```python
from build123d import *

# Parameters (mm, degrees)
F1_DEPTH = 8
F2_SIZE  = 30
F4_D     = 6.5
F6_D     = 10.5
F7_R     = 8
F8_R     = 3


with BuildPart() as f1:
    # F0 (on Front) → F1 (new body)
    with BuildSketch(Plane.XZ):
        Polygon((-41, 0), (0, 0), (0, 260), (-50, 260), (-50, 257), (-80, 257), (-80, 27), (-41, 27), align=None)
    extrude(amount=F1_DEPTH)

    # F2
    f2_edges = [f1.edges().sort_by_distance(p)[0] for p in [
        (0, -4, 260),
    ]]
    chamfer(f2_edges, length=F2_SIZE)

    # F4 (through all)
    with Locations(Plane.XZ.offset(8)):
        with Locations((-53, 176), (-68, 176), (-53, 126), (-68, 126), (-53, 76), (-68, 76)):
            Hole(F4_D / 2)

    # F6 (through all)
    with Locations(Plane.XZ.offset(8)):
        with Locations((-31.45, 249.2), (-31.45, 9.2)):
            Hole(F6_D / 2)

    # F7
    f7_edges = [f1.edges().sort_by_distance(p)[0] for p in [
        (-30, -4, 260),
        (0, -4, 230),
    ]]
    fillet(f7_edges, radius=F7_R)

    # F8
    f8_edges = [f1.edges().sort_by_distance(p)[0] for p in [
        (-41, -4, 27),
    ]]
    fillet(f8_edges, radius=F8_R)


solid = f1.part
```
Can you work these out from the model? Positions are in its coordinate system, mm. A direction names the side the tool comes from. Give positions to 0.01 mm unless a question says otherwise; leave off trailing zeros. Write each loop counter-clockwise with the first axis right and the second up, starting at its lowest first coordinate (ties: lowest second). Pieces come first, ordered by that corner, then holes. Notation, with made-up numbers: (41, 46) - (68, 46) arc R17 ccw to (68, 54) - close; hole circle Ø4 at (15, 55). An arc over 180 degrees is marked (long way). Write item = value, one per line. Start each with the question number.
1. Please list where these lines run through material, in increasing order: line 1 (X direction, y = -5.25, z = 176); line 2 (Z direction, x = -53, y = -2.5); line 3 (Z direction, x = -28.5, y = -6.25).
2. Imagine slicing it at A-A (z = 249.2). Please give me the cut outline in (x, y).
3. Imagine slicing it at C-C (x = -68). Please give me the cut outline in (y, z).
4. On a 3-axis mill with a long thin cutter (end or side, diameter ignored), from which of +Z, -Z, +X, -X, +Y, -Y can I reach the whole of each face in a straight line? I mean faces 4 (the face through (-65, -4, 257)), 5 (the face through (-30.767, -3.944, 254.405)), 6 (the face through (-41, -4, 12)). Say none if no direction works.
5. Imagine slicing it at D-D (z = 76). Please give me the cut outline in (x, y), and give its area (3 significant figures).
6. For pin 1 (4 mm diameter, centred on x = -57, y = -2.5, fed in from -Z); pin 2 (0.9 mm diameter, centred on y = -5, z = 258, fed in from -X); pin 3 (1 mm diameter, centred on x = -22, y = -6.5, fed in from +Z), each with a flat end and sliding along its axis, tell me the tip position at first contact or that it passes through.
7. Thinking about a two-plate mould opening in X: for faces 1 (the face through (-0.592, -4.056, 229.707)), 2 (the face through (-41, -8, 132)), 3 (the face through (-65.421, -3.944, 74.022)), which applies, released by +X, released by -X, zero draft, split by the parting line, or undercut?
8. Imagine slicing it at B-B (y = -2.25). Count the separate pieces of the cut face and the enclosed holes in it, and give its area (3 significant figures).
Worked answers:
q1.line_1 = -80 to -71.25, -64.75 to -56.25, -49.75 to 0
q1.line_2 = 27 to 72.75, 79.25 to 122.75, 129.25 to 172.75, 179.25 to 257
q1.line_3 = 0 to 4.86, 13.54 to 244.86, 253.54 to 258.39
q2.outline = (-80, -8) - (-36.7, -8) - (-36.7, 0) - (-80, 0) - close; (-26.2, -8) - (-19.2, -8) - (-19.2, 0) - (-26.2, 0) - close
q3.outline = (-8, 27) - (0, 27) - (0, 72.75) - (-8, 72.75) - close; (-8, 79.25) - (0, 79.25) - (0, 122.75) - (-8, 122.75) - close; (-8, 129.25) - (0, 129.25) - (0, 172.75) - (-8, 172.75) - close; (-8, 179.25) - (0, 179.25) - (0, 257) - (-8, 257) - close
q4.face_4 = +Z, -X, +Y, -Y
q4.face_5 = +Y, -Y
q4.face_6 = -Z, -X, +Y, -Y
q5.outline = (-80, -8) - (-71.25, -8) - (-71.25, 0) - (-80, 0) - close; (-64.75, -8) - (-56.25, -8) - (-56.25, 0) - (-64.75, 0) - close; (-49.75, -8) - (0, -8) - (0, 0) - (-49.75, 0) - close
q5.area = 536 mm2
q6.pin_1 = 27
q6.pin_2 = -50
q6.pin_3 = 252.5
q7.face_1 = released by +X
q7.face_2 = zero draft
q7.face_3 = undercut
q8.separate_pieces = 1
q8.enclosed_holes = 8
q8.area = 18,800 mm2
